from build123d import *

# Parameters (mm, degrees)
F_8_CLEARANCE_HOLE1_D     = 4.4958
F_8_CLEARANCE_HOLE1_DEPTH = 3.176
CIRPATTERN1_COUNT         = 6
SKETCH4_R                 = 88.9
CUT_EXTRUDE1_DEPTH        = 13.7


with BuildPart() as part:
    # Sketch1 → Revolve1 (revolve)
    with BuildSketch(Plane(origin=(0, 0, 0), x_dir=(0, 0, -1), z_dir=(1, 0, 0))):
        Polygon((89.535, 0), (92.71, 0), (92.71, 9.525), (124.46, 9.525), (124.46, 12.7), (0, 12.7), (0, 9.525), (89.535, 9.525), align=None)
    revolve(axis=Axis((0, 0, 0), (0, 1, 0)))

    # #8 Clearance Hole1
    with Locations(Plane(origin=(0, 12.7, 0), x_dir=(1, 0, 0), z_dir=(0, 1, 0))):
        with Locations((0, 114.3)):
            f_8_clearance_hole1 = Hole(F_8_CLEARANCE_HOLE1_D / 2, depth=F_8_CLEARANCE_HOLE1_DEPTH)

    # CirPattern1: #8 Clearance Hole1 ×6 about axis
    cirpattern1_axis = Axis((0, 0, 0), (0, 1, 0))
    for i in range(1, CIRPATTERN1_COUNT):
        add(f_8_clearance_hole1.rotate(cirpattern1_axis, i * 360 / CIRPATTERN1_COUNT), mode=Mode.SUBTRACT)

    # Sketch4 → Cut-Extrude1 (cut, through all)
    with BuildSketch(Plane(origin=(0, 12.7, 0), x_dir=(1, 0, 0), z_dir=(0, 1, 0))):
        Circle(SKETCH4_R)
    extrude(amount=-CUT_EXTRUDE1_DEPTH, mode=Mode.SUBTRACT)


solid = part.part
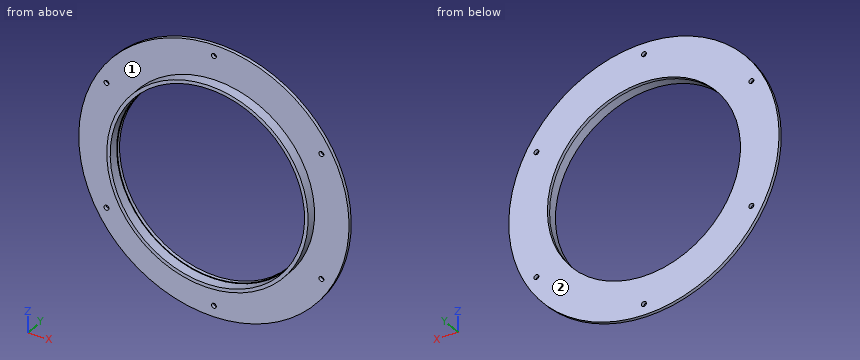
Can you work these out from the model? Positions are in its coordinate system, mm. Face numbers are marked on the shaded views. A direction names the side the tool comes from. Coordinates: 2 decimals unless noted, no trailing zeros. Write each loop counter-clockwise with the first axis right and the second up, starting at its lowest first coordinate (ties: lowest second). Pieces come first, ordered by that corner, then holes.
Q1. Please list where these lines run through material, in increasing order: L1, parallel to Z at x = 0, y = 10.9; L2, parallel to Z at x = 0, y = 4 (3 decimals).
Results found:
L1: z = -124.46 to -116.55, -112.05 to -88.9, 88.9 to 112.05, 116.55 to 124.46
L2: z = -92.71 to -89.535, 89.535 to 92.71
Q2. Imagine slicing it at D-D, the plane x = -107. List the corners of the cut face in (y, z) for me (3 decimals), plus the area to 3 significant figures.
Results found:
outline: (9.525, -63.571) - (12.7, -63.571) - (12.7, 63.571) - (9.525, 63.571) - close
area: 404 mm2
Q3. Imagine slicing it at A-A, the plane z = 0. List the corners of the cut face in (x, y) for me (3 decimals), plus the area to 3 significant figures.
Results found:
outline: (-124.46, 9.525) - (-92.71, 9.525) - (-92.71, 0) - (-89.535, 0) - (-89.535, 9.525) - (-88.9, 9.525) - (-88.9, 12.7) - (-124.46, 12.7) - close; (88.9, 9.525) - (89.535, 9.525) - (89.535, 0) - (92.71, 0) - (92.71, 9.525) - (124.46, 9.525) - (124.46, 12.7) - (88.9, 12.7) - close
area: 286 mm2
Q4. Imagine slicing it at C-C, the plane y = 6. List the corners of the cut face in (x, z) for me (3 decimals), plus the area to 3 significant figures.
Results found:
outline: circle Ø185.42 at (0, 0); hole circle Ø179.07 at (0, 0)
area: 1,820 mm2
Q5. Imagine slicing it at B-B, the plane x = -25.5. List the corners of the cut face in (y, z) for me (3 decimals).
Results found:
outline: (0, -89.134) - (9.525, -89.134) - (9.525, -121.82) - (12.7, -121.82) - (12.7, -85.164) - (9.525, -85.164) - (9.525, -85.827) - (0, -85.827) - close; (0, 85.827) - (9.525, 85.827) - (9.525, 85.164) - (12.7, 85.164) - (12.7, 121.82) - (9.525, 121.82) - (9.525, 89.134) - (0, 89.134) - close
Q6. Which directions (+Z, -Z, +X, -X, +Y, -Y) give clear straight access to the entire face, cutting with the end or side of a thin tool? Please do the marked faces 1 and 2.
Results found:
face 1: -Y
face 2: +Z, -Z, +X, -X, +Y
Q7. For P1, Ø1, axis at x = -51.5, y = 6.5, coming from the -Z side; P2, Ø2, axis at x = -98, y = 9, coming from the +Z side; P3, Ø7, axis at x = -98.99, z = 57.15, coming from the -Y side (3 decimals), each with a flat end and sliding along its axis, tell me the tip position at first contact or that it passes through.
Results found:
P1: stops at z = -77.42
P2: stops at z = 77.8
P3: stops at y = 9.525
